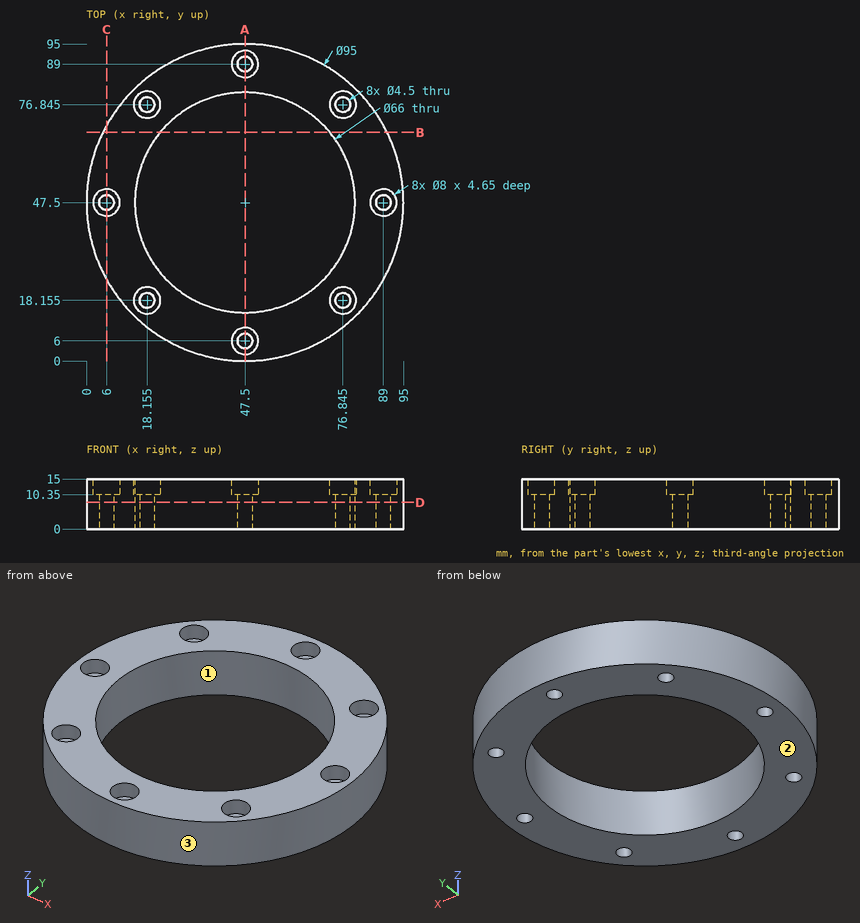
Check sheet for the drawn part. Datum: minimum x, y, z corner. Units: mm. Round coordinates to 2 decimals unless told otherwise and drop trailing zeros. Loops run counter-clockwise (first coordinate to the right, second up) from the corner with the lowest first, then second, coordinate; pieces in that order, holes last. Notation, with made-up numbers: (-2.75, 38) - (49.25, 38) arc R29 ccw to (49.25, 74) - close; hole circle Ø3 at (74, -9.5). An arc over 180 degrees is marked (long way). Write each question's results on one line, items separated by ' | '. Start each with the question number.
Q1. Gauge pin test, flat ends, axial feed: P1, Ø5, axis at x = 6, y = 47.5, coming from the +Z side; P2, Ø2, axis at y = 73, z = 1.5, coming from the +X side; P3, Ø2, axis at y = 10.5, z = 5, coming from the +X side. Record the tip position at first contact, or that the pin passes through.
Q2. Thickness scan on line 1 (Y direction, x = 47.5, z = 6.5); line 2 (Y direction, x = 49, z = 7); line 3 (X direction, y = 23, z = 12.75). Record the ranges inside material, lowest first. Write a range as [from, to].
Q3. Cross-section at A-A on x = 47.5. Enter the section's corners in (y, z).
Q4. Cross-section at D-D on z = 8. State how many separate pieces and enclosed holes the cut face has, and give its area (3 significant figures).
Q5. Cross-section at C-C on x = 6. Enter the section's corners in (y, z).
Q6. Release check for a two-part mould opening along Y. For the marked faces 1, 2 and 3 record: +Y half, -Y half, draft (parallel to the pull), parting line (faces both ways), or undercut.
Q7. Cross-section at B-B on y = 68.5. Enter the section's corners in (x, z).
Answers below:
1) P1: stops at z = 10.35 | P2: stops at x = 88.19 | P3: stops at x = 78.49
2) line 1: y = [0, 3.75], [8.25, 14.5], [80.5, 86.75], [91.25, 95] | line 2: y = [0.02, 4.32], [7.68, 14.53], [80.47, 87.32], [90.68, 94.98] | line 3: x = [6.81, 25.39], [69.61, 88.19]
3) outline: (0, 0) - (3.75, 0) - (3.75, 10.35) - (2, 10.35) - (2, 15) - (0, 15) - close; (8.25, 0) - (14.5, 0) - (14.5, 15) - (10, 15) - (10, 10.35) - (8.25, 10.35) - close; (80.5, 0) - (86.75, 0) - (86.75, 10.35) - (85, 10.35) - (85, 15) - (80.5, 15) - close; (91.25, 0) - (95, 0) - (95, 15) - (93, 15) - (93, 10.35) - (91.25, 10.35) - close
4) separate pieces: 1 | enclosed holes: 9 | area: 3,540 mm²
5) outline: (24.39, 0) - (45.25, 0) - (45.25, 10.35) - (43.5, 10.35) - (43.5, 15) - (24.39, 15) - close; (49.75, 0) - (70.61, 0) - (70.61, 15) - (51.5, 15) - (51.5, 10.35) - (49.75, 10.35) - close
6) face 1: undercut | face 2: draft | face 3: parting line
7) outline: (4.89, 0) - (22.04, 0) - (22.04, 15) - (4.89, 15) - close; (72.96, 0) - (90.11, 0) - (90.11, 15) - (72.96, 15) - close
